Geometry check sheet. Reference: the model listing, model coordinates, mm. Face numbers are marked on the shaded views. A direction names the side the tool comes from. Coordinates: 2 decimals unless noted, no trailing zeros. Loops run counter-clockwise (first coordinate to the right, second up) from the corner with the lowest first, then second, coordinate; pieces in that order, holes last.
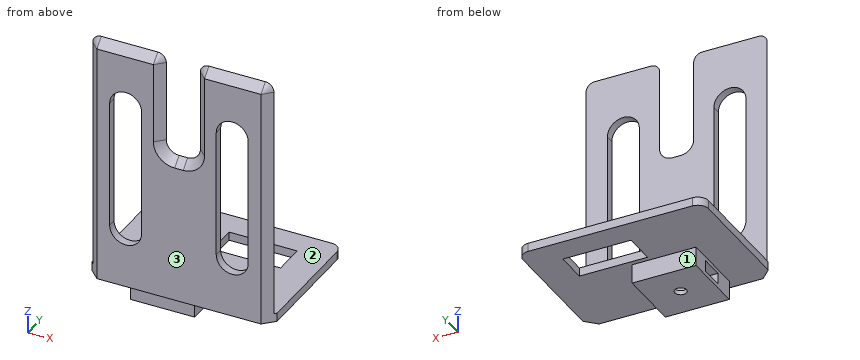
from build123d import *

# Parameters (mm, degrees)
F1_DEPTH      = 4
F2_W          = 87
F2_H          = 4
F3_DEPTH      = 60
F4_W          = 32
F4_H          = 15
F5_DEPTH      = 4
F6_R          = 5
F7_W          = 30
F7_H          = 30
F7_R          = 2.75
F8_DEPTH      = 9
F9_DEPTH      = 5
F10_T1_DEPTH  = 26.5
F10_T3_DEPTH  = 125.8584149398
F10_T5_DEPTH  = 38
F10_T7_DEPTH  = 4
F10_T9_DEPTH  = 26.5
F10_T12_ANGLE = 90
F10_T14_ANGLE = 90
F10_T16_ANGLE = 90
F10_T18_ANGLE = 90
F10_T20_ANGLE = 90
F10_T22_ANGLE = 90
F11_W         = 11.3
F11_H         = 5.2
F12_DEPTH     = 30.7


# Not quite as in the source:
# - a fillet or chamfer that OpenCascade refuses, or shapes differently, is made with other operations: its cross-section is extruded or revolved along the edge and cut away or added


with BuildPart() as f1:
    # F0 (on Front) → F1 (new body)
    with BuildSketch(Plane.XZ):
        Polygon((-7, 78.3899563551), (-43.5, 78.3899563551), (-43.5, -39.6100436449), (43.5, -39.6100436449), (43.5, 78.3899563551), (7, 78.3899563551), (7, 30.3899563551), (-7, 30.3899563551), align=None)
        with BuildLine():
            Line((-17.5, 48.3899563551), (-17.5, -11.6100436449))
            ThreePointArc((-17.5, -11.6100436449), (-25, -19.1100436449), (-32.5, -11.6100436449))
            Line((-32.5, -11.6100436449), (-32.5, 48.3899563551))
            ThreePointArc((-32.5, 48.3899563551), (-25, 55.8899563551), (-17.5, 48.3899563551))
        make_face(mode=Mode.SUBTRACT)
        with BuildLine():
            Line((32.5, 48.3899563551), (32.5, -11.6100436449))
            ThreePointArc((32.5, -11.6100436449), (25, -19.1100436449), (17.5, -11.6100436449))
            Line((17.5, -11.6100436449), (17.5, 48.3899563551))
            ThreePointArc((17.5, 48.3899563551), (25, 55.8899563551), (32.5, 48.3899563551))
        make_face(mode=Mode.SUBTRACT)
    extrude(amount=F1_DEPTH)

    # F2 (on face) → F3 (join)
    with BuildSketch(Plane(origin=(0, 0, 0), x_dir=(-1, 0, 0), z_dir=(0, 1, 0))):
        with Locations((0, -37.6100436449)):
            Rectangle(F2_W, F2_H)
    extrude(amount=F3_DEPTH)

    # F4 (on face) → F5 (cut)
    with BuildSketch(Plane(origin=(0, 0, -39.6100436449), x_dir=(1, 0, 0), z_dir=(0, 0, -1))):
        with Locations((12.5, -40.5)):
            Rectangle(F4_W, F4_H)
    extrude(amount=-F5_DEPTH, mode=Mode.SUBTRACT)

    # F6
    f6_edges = [f1.edges().sort_by_distance(p)[0] for p in [
        (-43.5, -2, 78.389956),
        (7, -2, 78.389956),
        (-7, -2, 78.389956),
        (43.5, -2, 78.389956),
        (-43.5, 60, -37.610044),
        (43.5, 60, -37.610044),
        (7, -2, 30.389956),
        (-7, -2, 30.389956),
    ]]
    fillet(f6_edges, radius=F6_R)

    # F7 (on face) → F8 (join)
    with BuildSketch(Plane(origin=(0, 0, -39.6100436449), x_dir=(1, 0, 0), z_dir=(0, 0, -1))):
        with Locations((-10.0618535653, -15.7216744063)):
            Rectangle(F7_W, F7_H)
        with Locations((-10.0618535653, -15.7216744063)):
            Circle(F7_R, mode=Mode.SUBTRACT)
    extrude(amount=F8_DEPTH)

    # F9 (cut): a face of the model
    f9_faces = [f1.faces().sort_by_distance(p)[0] for p in [
        (-10.0618535653, 15.7216744063, -39.6100436449),
    ]]
    extrude(f9_faces, amount=-F9_DEPTH, mode=Mode.SUBTRACT)

    # F10: chamfer of 5 on 1 edges, made by hand

    # F10_s2 → F10_t1 (cut)
    with BuildSketch(Plane.YZ.offset(-38.5)):
        Polygon((-4, 73.3899563551), (1, 78.3899563551), (-4, 78.3899563551), align=None)
    extrude(amount=F10_T1_DEPTH, mode=Mode.SUBTRACT)

    # F10_s4 → F10_t3 (cut)
    with BuildSketch(Plane.XY.offset(-52.4684585847)):
        Polygon((-38.5, -4), (-43.5, 1), (-43.5, -4), align=None)
        Polygon((38.5, -4), (43.5, 1), (43.5, -4), align=None)
    extrude(amount=F10_T3_DEPTH, mode=Mode.SUBTRACT)

    # F10_s6 → F10_t5 (cut)
    with BuildSketch(Plane.XY.offset(35.3899563551)):
        Polygon((-7, 1), (-12, -4), (-7, -4), align=None)
        Polygon((12, -4), (7, 1), (7, -4), align=None)
    extrude(amount=F10_T5_DEPTH, mode=Mode.SUBTRACT)

    # F10_s8 → F10_t7 (cut)
    with BuildSketch(Plane.YZ.offset(-2)):
        Polygon((-4, 25.3899563551), (1, 30.3899563551), (-4, 30.3899563551), align=None)
    extrude(amount=F10_T7_DEPTH, mode=Mode.SUBTRACT)

    # F10_s10 → F10_t9 (cut)
    with BuildSketch(Plane.YZ.offset(12)):
        Polygon((-4, 73.3899563551), (1, 78.3899563551), (-4, 78.3899563551), align=None)
    extrude(amount=F10_T9_DEPTH, mode=Mode.SUBTRACT)

    # F10_s11 → F10_t12 (revolve, cut)
    with BuildSketch(Plane.XY.offset(73.3899563551)):
        Polygon((-7, 1), (-12, -4), (-7, -4), align=None)
    revolve(axis=Axis((-12, -4, 73.3899563551), (0, -1, 0)), revolution_arc=F10_T12_ANGLE, mode=Mode.SUBTRACT)

    # F10_s13 → F10_t14 (revolve, cut)
    with BuildSketch(Plane.YZ.offset(-38.5)):
        Polygon((-4, 73.3899563551), (1, 78.3899563551), (-4, 78.3899563551), align=None)
    revolve(axis=Axis((-38.5, -4, 73.3899563551), (0, -1, 0)), revolution_arc=F10_T14_ANGLE, mode=Mode.SUBTRACT)

    # F10_s15 → F10_t16 (revolve, cut)
    with BuildSketch(Plane.XY.offset(35.3899563551)):
        Polygon((-7, 1), (-12, -4), (-7, -4), align=None)
    revolve(axis=Axis((-2, -4, 35.3899563551), (0, -1, 0)), revolution_arc=F10_T16_ANGLE, mode=Mode.SUBTRACT)

    # F10_s17 → F10_t18 (revolve, cut)
    with BuildSketch(Plane.YZ.offset(2)):
        Polygon((-4, 25.3899563551), (1, 30.3899563551), (-4, 30.3899563551), align=None)
    revolve(axis=Axis((2, -4, 35.3899563551), (0, -1, 0)), revolution_arc=F10_T18_ANGLE, mode=Mode.SUBTRACT)

    # F10_s19 → F10_t20 (revolve, cut)
    with BuildSketch(Plane.XY.offset(73.3899563551)):
        Polygon((12, -4), (7, 1), (7, -4), align=None)
    revolve(axis=Axis((12, -4, 73.3899563551), (0, 1, 0)), revolution_arc=F10_T20_ANGLE, mode=Mode.SUBTRACT)

    # F10_s21 → F10_t22 (revolve, cut)
    with BuildSketch(Plane.YZ.offset(38.5)):
        Polygon((-4, 73.3899563551), (1, 78.3899563551), (-4, 78.3899563551), align=None)
    revolve(axis=Axis((38.5, -4, 73.3899563551), (0, 1, 0)), revolution_arc=F10_T22_ANGLE, mode=Mode.SUBTRACT)

    # F11 (on face) → F12 (cut)
    with BuildSketch(Plane.YZ.offset(4.9381464347)):
        with Locations((16.5075063076, -44.0100436449)):
            Rectangle(F11_W, F11_H)
    extrude(amount=-F12_DEPTH, mode=Mode.SUBTRACT)


solid = f1.part
(1) Sectioned sample at B-B on x = 25. Record the cut outline in (y, z).
Findings:
outline: (-4, -39.61) - (33, -39.61) - (33, -35.61) - (0, -35.61) - (0, -19.11) - (-4, -19.11) - close; (-4, 55.89) - (0, 55.89) - (0, 77.39) - (-4, 73.39) - close; (48, -39.61) - (60, -39.61) - (60, -35.61) - (48, -35.61) - close
(2) Scan lines: L1, parallel to Z at x = -11, y = 20.5; L2, parallel to Y at x = 34.5, z = 65.5; L3, parallel to Z at x = -37, y = 37.5. Record each from-to range of solid material in increasing order.
Findings:
L1: z = -48.61 to -46.61, -41.41 to -35.61
L2: y = -4 to 0
L3: z = -39.61 to -35.61
(3) Access from +Z, -Z, +X, -X, +Y, -Y to the whole of each face (thin tool, end or side, straight path). Record for the marked faces 1, 2 and 3.
Findings:
face 1: -Z, +X, -X, +Y
face 2: +Z, +X, -X, +Y
face 3: +Z, -Z, +X, -X, -Y
(4) Sectioned sample at A-A on y = 34.5. Record the cut outline in (x, z).
Findings:
outline: (-43.5, -39.61) - (-3.5, -39.61) - (-3.5, -35.61) - (-43.5, -35.61) - close; (28.5, -39.61) - (43.5, -39.61) - (43.5, -35.61) - (28.5, -35.61) - close
(5) Sectioned sample at C-C on z = 50. Record the cut outline in (x, y), and give its area (3 significant figures).
Findings:
outline: (-42.5, 0) - (-38.5, -4) - (-32.33, -4) - (-32.33, 0) - close; (-17.67, -4) - (-12, -4) - (-8, 0) - (-17.67, 0) - close; (8, 0) - (12, -4) - (17.67, -4) - (17.67, 0) - close; (32.33, -4) - (38.5, -4) - (42.5, 0) - (32.33, 0) - close
area: 127 mm2
(6) Gauge pin test, flat ends, axial feed: pin 1 Ø2 at (y, z) = (-1.5, 21.5) entering from +X; pin 2 Ø2 at (x, y) = (-22.5, 7.5) entering from +Z; pin 3 Ø4.5 at (y, z) = (-1, 22.5) entering from +X; pin 4 Ø5 at (x, y) = (-10.06, 15.72) entering from -Z. Record the tip position at first contact, or that the pin passes through.
Findings:
pin 1: stops at x = 42
pin 2: stops at z = -35.61
pin 3: stops at x = 42.5
pin 4: passes through
(7) Sectioned sample at D-D on x = 34. Record the cut outline in (y, z), and give its area (3 significant figures).
Findings:
outline: (-4, -39.61) - (60, -39.61) - (60, -35.61) - (0, -35.61) - (0, 77.39) - (-4, 73.39) - close
area: 700 mm2
